The model under review builds one solid part; all positions refer to its coordinate system, in mm. Face numbers are marked on the shaded views. A direction names the side the tool comes from. Give positions to 0.01 mm unless a question says otherwise; leave off trailing zeros. Order: outer loops, then holes, each group sorted by start corner. A loop starts at its lowest first (then second) coordinate and runs counter-clockwise, first axis right, second up. Notation, with made-up numbers: (18.5, 18.5) - (71.5, 18.5) arc R13 ccw to (71.5, 34.5) - close; hole circle Ø8 at (-24, 55). An arc over 180 degrees is marked (long way). Answer as CSV lines item,"result". Start each with the question number.
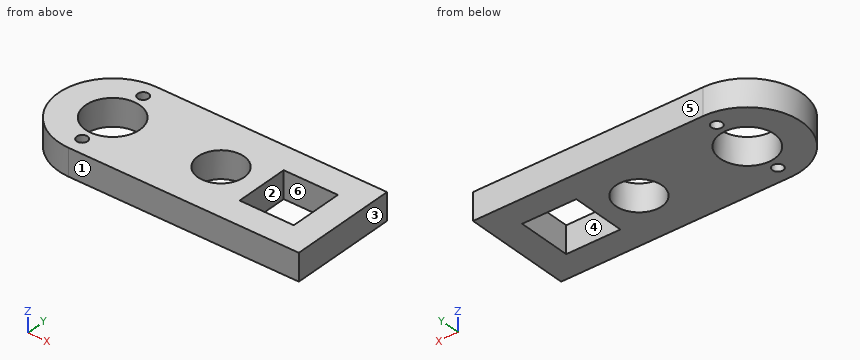
from build123d import *

# Parameters (mm, degrees)
SKETCH1_R           = 4.25
SKETCH1_R_2         = 5
SKETCH1_R_3         = 1
BOSS_EXTRUDE1_DEPTH = 5
SKETCH2_R           = 1
SKETCH2_R_2         = 1.224011965
BOSS_EXTRUDE2_DEPTH = 5


with BuildPart() as part:
    # Sketch1 → Boss-Extrude1 (new body)
    with BuildSketch(Plane.XY):
        with BuildLine():
            Line((0, 10), (42.5, 10))
            Line((42.5, 10), (42.5, -10))
            Line((42.5, -10), (0, -10))
            ThreePointArc((0, -10), (-10, 0), (0, 10))
        make_face()
        with Locations((20, 0)):
            Circle(SKETCH1_R, mode=Mode.SUBTRACT)
        Circle(SKETCH1_R_2, mode=Mode.SUBTRACT)
        with Locations((7, 0.062454575)):
            Circle(SKETCH1_R_3, mode=Mode.SUBTRACT)
        with Locations((0.062454575, -7)):
            Circle(SKETCH1_R_3, mode=Mode.SUBTRACT)
        with Locations((-7, -0.062454575)):
            Circle(SKETCH1_R_3, mode=Mode.SUBTRACT)
        with Locations((-0.062454575, 7)):
            Circle(SKETCH1_R_3, mode=Mode.SUBTRACT)
        Polygon((27.5, 5), (32.5, 5), (37.5, 5), (37.5, -5), (32.5, -5), (27.5, -5), (27.5, 0), align=None, mode=Mode.SUBTRACT)
    extrude(amount=BOSS_EXTRUDE1_DEPTH)

    # Sketch2 → Boss-Extrude2 (add)
    with BuildSketch(Plane(origin=(0, 0, 0), x_dir=(-1, 0, 0), z_dir=(0, 0, -1))):
        with Locations((7, -0.062454575)):
            Circle(SKETCH2_R)
        with Locations((-7, 0.062454575)):
            Circle(SKETCH2_R_2)
    extrude(amount=-BOSS_EXTRUDE2_DEPTH)


solid = part.part
Item 1: Machinability: for the marked faces 1 and 2, which of the approach directions +Z, -Z, +X, -X, +Y, -Y give a long, thin tool a straight path to every point of the face, cutting with its end or side? Answer none if there is none.
Item 2: Take a section at B-B on x = 20. Write out the cut boundary in (y, z), and give its area (3 significant figures).
Item 3: Take a section at D-D on y = 7. Write out the cut boundary in (x, z).
Item 4: Take a section at A-A on y = 0. Write out the cut boundary in (x, z).
Item 5: Mouldability with a two-part tool opening along X and no side actions: class the marked faces 3, 4, 5 and 6 as released by +X, released by -X, zero draft, split by the parting line, or undercut.
Item 6: Clearance check with a flat-ended pin moving along its axis: pin 1 (7.5 mm diameter, centred on x = 20, y = 0, fed in from -Z). State where the tip first meets the part, or that it passes through.
Item 7: Take a section at C-C on z = 0.65. Write out the cut boundary in (x, y).
Item 8: For line 1 along Y through (x, z) = (0, 1); line 2 along X through (y, z) = (0.25, 2.95); line 3 along Y through (x, z) = (34.5, 3.7), list the stretches that pass through material, from the lowest coordinate up.
Data:
1,face 1,"+Z, -Z, +X, -X, -Y"
1,face 2,"+Z, -Z"
2,outline,"(-10, 0) - (-4.25, 0) - (-4.25, 5) - (-10, 5) - close; (4.25, 0) - (10, 0) - (10, 5) - (4.25, 5) - close"
2,area,"57.5 mm^2"
3,outline,"(-7.14, 0) - (-1.06, 0) - (-1.06, 5) - (-7.14, 5) - close; (0.94, 0) - (42.5, 0) - (42.5, 5) - (0.94, 5) - close"
4,outline,"(-10, 0) - (-5, 0) - (-5, 5) - (-10, 5) - close; (5, 0) - (15.75, 0) - (15.75, 5) - (5, 5) - close; (24.25, 0) - (27.5, 0) - (27.5, 5) - (24.25, 5) - close; (37.5, 0) - (42.5, 0) - (42.5, 5) - (37.5, 5) - close"
5,face 3,"released by +X"
5,face 4,"undercut"
5,face 5,"zero draft"
5,face 6,"undercut"
6,pin 1,"passes through"
7,outline,"(0, -10) - (42.5, -10) - (42.5, 10) - (0, 10) arc R10 ccw to start; hole circle Ø10 at (0, 0); hole circle Ø2 at (-0.06, 7); hole circle Ø2 at (0.06, -7); hole circle Ø8.5 at (20, 0); hole (27.5, -5) - (37.5, -5) - (37.5, 5) - (27.5, 5) - close"
8,line 1,"y = -10 to -8, -6 to -5, 5 to 6, 8 to 10"
8,line 2,"x = -10 to -4.99, 4.99 to 15.76, 24.24 to 27.5, 37.5 to 42.5"
8,line 3,"y = -10 to -5, 5 to 10"
